Part model, mm, in its own coordinate system. A direction names the side the tool comes from. Coordinates: 2 decimals unless noted, no trailing zeros. Order: outer loops, then holes, each group sorted by start corner. A loop starts at its lowest first (then second) coordinate and runs counter-clockwise, first axis right, second up.
from build123d import *

# Parameters (mm, degrees)
SKETCH_1_W          = 35
SKETCH_1_H          = 35
SKETCH_1_R          = 1.5
SKETCH_1_W_2        = 25
SKETCH_1_H_2        = 18
EXTRUDE_2_DEPTH     = 4
SKETCH_2_W          = 15
SKETCH_2_H          = 9
CUT_EXTRUDE_1_DEPTH = 4
SKETCH_3_W          = 35
SKETCH_3_H          = 4
EXTRUDE_3_DEPTH     = 4
SKETCH_4_W          = 4
SKETCH_4_H          = 39
EXTRUDE_4_DEPTH     = 9
SKETCH_5_W          = 4
SKETCH_5_H          = 39
EXTRUDE_5_DEPTH     = 9
SKETCH_6_W          = 4
SKETCH_6_H          = 39
EXTRUDE_6_DEPTH     = 30
CUT_EXTRUDE_2_REACH = 80.946
SKETCH_7_R          = 1.5
CUT_EXTRUDE_3_REACH = 80.946


with BuildPart() as part:
    # 草图1 → 凸台-拉伸2 (new body)
    with BuildSketch(Plane.XY):
        with Locations((-93.185913744, 26.117851257)):
            Rectangle(SKETCH_1_W, SKETCH_1_H)
        with Locations((-106.435913744, 39.367851257)):
            Circle(SKETCH_1_R, mode=Mode.SUBTRACT)
        with Locations(Location((-79.935913744, 12.867851257, 0), (0, 0, 180))):
            Circle(SKETCH_1_R, mode=Mode.SUBTRACT)
        with Locations((-79.935913744, 39.367851257)):
            Circle(SKETCH_1_R, mode=Mode.SUBTRACT)
        with Locations(Location((-106.435913744, 12.867851257, 0), (0, 0, 180))):
            Circle(SKETCH_1_R, mode=Mode.SUBTRACT)
        with Locations((-93.185913744, 26.117851257)):
            Rectangle(SKETCH_1_W_2, SKETCH_1_H_2, mode=Mode.SUBTRACT)
    extrude(amount=EXTRUDE_2_DEPTH)

    # 草图2 → 切除-拉伸1 (cut)
    with BuildSketch(Plane.XY.offset(4)):
        with Locations((-93.185913744, 39.117851257)):
            Rectangle(SKETCH_2_W, SKETCH_2_H)
    extrude(amount=-CUT_EXTRUDE_1_DEPTH, mode=Mode.SUBTRACT)

    # 草图3 → 凸台-拉伸3 (add)
    with BuildSketch(Plane(origin=(0, 43.617851257, 0), x_dir=(1, 0, 0), z_dir=(0, 1, 0))):
        with Locations((-93.185913744, -2)):
            Rectangle(SKETCH_3_W, SKETCH_3_H)
    extrude(amount=EXTRUDE_3_DEPTH)

    # 草图4 → 凸台-拉伸4 (add)
    with BuildSketch(Plane(origin=(-75.685913744, 0, 0), x_dir=(0, 0, -1), z_dir=(1, 0, 0))):
        with Locations((-2, 28.117851257)):
            Rectangle(SKETCH_4_W, SKETCH_4_H)
    extrude(amount=EXTRUDE_4_DEPTH)

    # 草图5 → 凸台-拉伸5 (add)
    with BuildSketch(Plane.ZY.offset(110.685913744)):
        with Locations((2, 28.117851257)):
            Rectangle(SKETCH_5_W, SKETCH_5_H)
    extrude(amount=EXTRUDE_5_DEPTH)

    # 草图6 → 凸台-拉伸6 (add)
    with BuildSketch(Plane.XY.offset(4)):
        with Locations((-117.685913744, 28.117851257)):
            Rectangle(SKETCH_6_W, SKETCH_6_H)
        with Locations((-68.685913744, 28.117851257)):
            Rectangle(SKETCH_6_W, SKETCH_6_H)
    extrude(amount=EXTRUDE_6_DEPTH)

    # 切除-拉伸2: up to this face of the body (flat: up to its plane)
    cut_extrude_2_end = Plane(part.part.faces().sort_by_distance((-66.685913744, 28.117851257, 17))[0])
    # 草图7 → 切除-拉伸2 (cut, up to the picked face)
    with BuildSketch(Plane.ZY.offset(119.685913744), mode=Mode.PRIVATE) as cut_extrude_2_sk1:
        with Locations(Location((24, 28.117851257, 0), (0, 0, 90))):
            Circle(SKETCH_7_R)
    cut_extrude_2_tool1 = split(extrude(cut_extrude_2_sk1.sketch, amount=-CUT_EXTRUDE_2_REACH, mode=Mode.PRIVATE), bisect_by=cut_extrude_2_end, keep=Keep.BOTH, mode=Mode.PRIVATE)
    add(cut_extrude_2_tool1.solids().sort_by(Axis((-119.685914, 28.117851, 24), (1, 0, 0)))[0], mode=Mode.SUBTRACT)

    # 切除-拉伸3: up to this face of the body (flat: up to its plane)
    cut_extrude_3_end = Plane(part.part.faces().sort_by_distance((-66.685913744, 28.117851257, 16.962484718))[0])
    # 草图9 → 切除-拉伸3 (cut, up to the picked face)
    with BuildSketch(Plane.ZY.offset(119.685913744), mode=Mode.PRIVATE) as cut_extrude_3_sk1:
        with BuildLine():
            Line((34, 44.8585203), (34, 47.617851257))
            Line((34, 47.617851257), (24, 47.617851257))
            ThreePointArc((24, 47.617851257), (29.186856161, 46.915365007), (34, 44.8585203))
        make_face()
    cut_extrude_3_tool1 = split(extrude(cut_extrude_3_sk1.sketch, amount=-CUT_EXTRUDE_3_REACH, mode=Mode.PRIVATE), bisect_by=cut_extrude_3_end, keep=Keep.BOTH, mode=Mode.PRIVATE)
    # 草图9 → 切除-拉伸3 (cut, up to the picked face)
    with BuildSketch(Plane.ZY.offset(119.685913744), mode=Mode.PRIVATE) as cut_extrude_3_sk2:
        with BuildLine():
            ThreePointArc((34, 11.377182214), (29.186856161, 9.320337507), (24, 8.617851257))
            Line((24, 8.617851257), (34, 8.617851257))
            Line((34, 8.617851257), (34, 11.377182214))
        make_face()
    cut_extrude_3_tool2 = split(extrude(cut_extrude_3_sk2.sketch, amount=-CUT_EXTRUDE_3_REACH, mode=Mode.PRIVATE), bisect_by=cut_extrude_3_end, keep=Keep.BOTH, mode=Mode.PRIVATE)
    add(cut_extrude_3_tool1.solids().sort_by(Axis((-119.685914, 46.80116, 31.536753), (1, 0, 0)))[0], mode=Mode.SUBTRACT)
    add(cut_extrude_3_tool2.solids().sort_by(Axis((-119.685914, 9.434542, 31.536753), (1, 0, 0)))[0], mode=Mode.SUBTRACT)


solid = part.part
Q1. Cut at A-A on x = -89. Write the cut outline in (y, z), and give its area (3 significant figures).
Results list:
outline: (8.62, 0) - (17.12, 0) - (17.12, 4) - (8.62, 4) - close; (43.62, 0) - (47.62, 0) - (47.62, 4) - (43.62, 4) - close
area: 50.0 mm2
Q2. Cut at B-B on z = 12. Write the cut outline in (x, y).
Results list:
outline: (-119.69, 8.62) - (-115.69, 8.62) - (-115.69, 47.62) - (-119.69, 47.62) - close; (-70.69, 8.62) - (-66.69, 8.62) - (-66.69, 47.62) - (-70.69, 47.62) - close
Q3. Cut at D-D on y = 42. Write the cut outline in (x, z), and give its area (3 significant figures).
Results list:
outline: (-119.69, 0) - (-100.69, 0) - (-100.69, 4) - (-115.69, 4) - (-115.69, 34) - (-119.69, 34) - close; (-85.69, 0) - (-66.69, 0) - (-66.69, 34) - (-70.69, 34) - (-70.69, 4) - (-85.69, 4) - close
area: 392 mm2
Q4. Mould opens along X. For faces 4 (the face through (-85.686, 39, 2)), 5 (the face through (-119.686, 28, 17)), 6 (the face through (-68.71, 9.34, 29.26)) say: pulls with the +X half, pulls with the -X half, needs draft (parallel to the pull), parting line crosses it, or undercut.
Results list:
face 4: undercut
face 5: pulls with the -X half
face 6: needs draft
Q5. Wall check: line 1 along X through (y, z) = (27, 1.5); line 2 along X through (y, z) = (11.5, 13.5); line 3 along Y through (x, z) = (-68, 24). Give the ranges that are in metal, low to high.
Results list:
line 1: x = -119.69 to -105.69, -80.69 to -66.69
line 2: x = -119.69 to -115.69, -70.69 to -66.69
line 3: y = 8.62 to 26.62, 29.62 to 47.62
Q6. Pin check, flat tips, straight feed: pin 1 Ø4 at (x, y) = (-79.94, 39.37) entering from -Z; pin 2 Ø10 at (x, z) = (-111.5, 30.5) entering from -Y; pin 3 Ø5 at (x, y) = (-106.44, 39.37) entering from +Z; pin 4 Ø1.8 at (y, z) = (28.12, 24) entering from +X. Stop position of each tip, or through.
Results list:
pin 1: stops at z = 0
pin 2: stops at y = 8.98
pin 3: stops at z = 4
pin 4: passes through
Q7. Which spindle directions (+Z, -Z, +X, -X, +Y, -Y) get a long thin tool onto all of the face, cutting with end or side? Do faces 1 (the face through (-100.686, 39, 2)), 2 (the face through (-118, 27, 23)), 3 (the face through (-93, 15, 4)). Say none if no direction does.
Results list:
face 1: +Z, -Z
face 2: +X, -X
face 3: +Z, +Y, -Y
Q8. Cut at C-C on y = 23.5. Write the cut outline in (x, z).
Results list:
outline: (-119.69, 0) - (-105.69, 0) - (-105.69, 4) - (-115.69, 4) - (-115.69, 34) - (-119.69, 34) - close; (-80.69, 0) - (-66.69, 0) - (-66.69, 34) - (-70.69, 34) - (-70.69, 4) - (-80.69, 4) - close
